Geometry: see drawing. Coordinates: mm, zero at the bounding-box minimum. A direction names the side the tool comes from. Round coordinates to 2 decimals unless told otherwise and drop trailing zeros. Write each loop counter-clockwise with the first axis right and the second up, starting at its lowest first coordinate (ties: lowest second). Pieces come first, ordered by that corner, then holes. Notation, with made-up numbers: (12, 48) -> (56, 48) arc R27 cw to (56, 72) -> close; hole circle Ø3 at (-36.5, -30). An arc over 180 degrees is marked (long way). Write item = value, one per line.
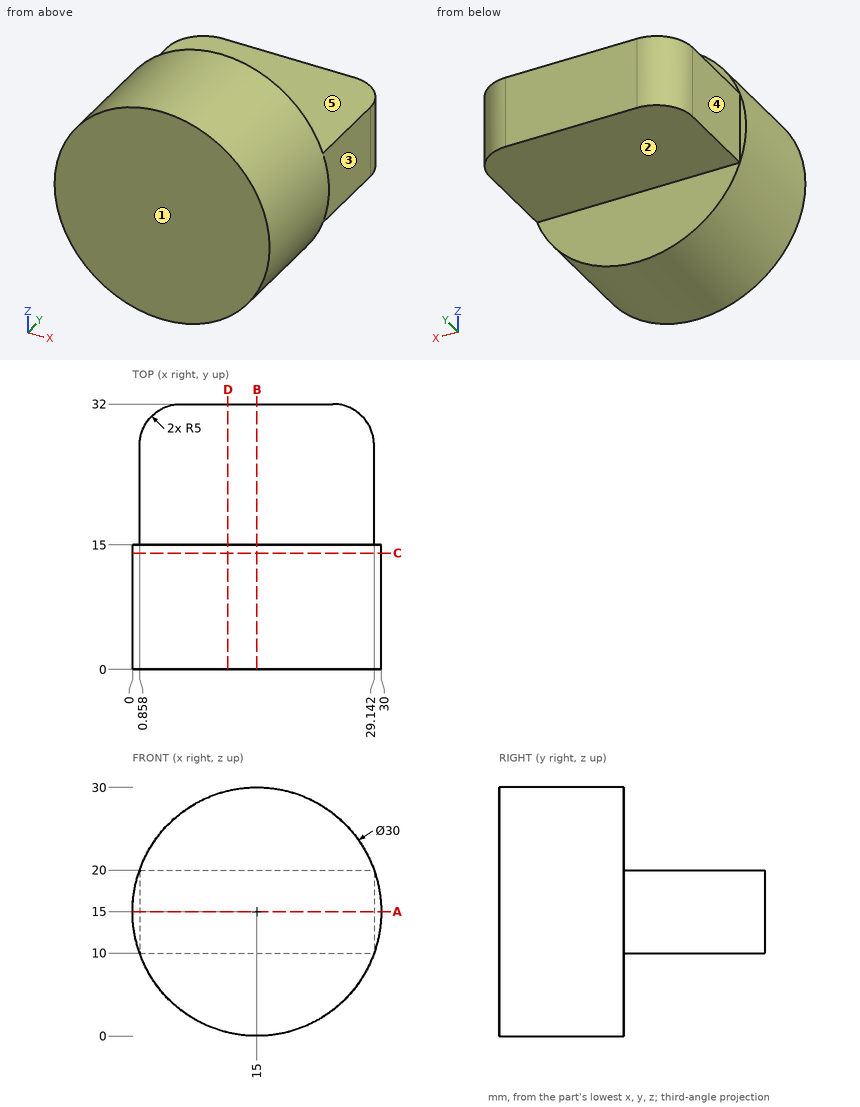
1) Cut plane A-A (z = 15). Return the cut outline in (x, y).
Solutions:
outline = (0, 0) -> (30, 0) -> (30, 15) -> (29.14, 15) -> (29.14, 27) arc R5 ccw to (24.14, 32) -> (5.86, 32) arc R5 ccw to (0.86, 27) -> (0.86, 15) -> (0, 15) -> close
2) Line query: L1, parallel to Y at x = 14.5, z = 21; L2, parallel to X at y = 23, z = 13.5; L3, parallel to Z at x = 14.75, y = 8. Output: solid intervals per line, ascending. Write a range as from..to.
Solutions:
L1 = 0..15
L2 = 0.86..29.14
L3 = 0..30
3) First-contact query: P1, Ø3, axis at x = 15, y = 19.5, coming from the -Z side; P2, Ø5, axis at y = 10.5, z = 26, coming from the -X side; P3, Ø1, axis at x = 26.5, y = 19, coming from the +Z side. Flat tips, straight axial feed; report the tip coordinate or a pass-through.
Solutions:
P1 = 10
P2 = 2.64
P3 = 20
4) Cut plane D-D (x = 11.5). Return the cut outline in (y, z).
Solutions:
outline = (0, 0.41) -> (15, 0.41) -> (15, 10) -> (32, 10) -> (32, 20) -> (15, 20) -> (15, 29.59) -> (0, 29.59) -> close
5) Cut plane B-B (x = 15). Return the cut outline in (y, z).
Solutions:
outline = (0, 0) -> (15, 0) -> (15, 10) -> (32, 10) -> (32, 20) -> (15, 20) -> (15, 30) -> (0, 30) -> close
6) Cut plane C-C (y = 14). Return the cut outline in (x, z), and give its area (3 significant figures).
Solutions:
outline = circle Ø30 at (15, 15)
area = 707 mm^2
7) Access query for the marked faces 1, 2, 3, 4 and 5. Directions: +Z, -Z, +X, -X, +Y, -Y. A direction counts if a zero-diameter tool reaches every point of the face in a straight line with its end or side. Return the directions, or none.
Solutions:
face_1 = +Z, -Z, +X, -X, -Y
face_2 = -Z, +X, -X, +Y
face_3 = +Z, -Z, +X, +Y
face_4 = +Z, -Z, -X, +Y
face_5 = +Z, +X, -X, +Y
